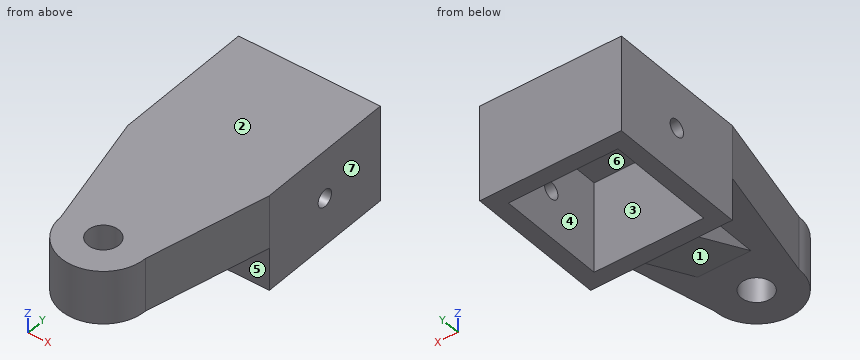
from build123d import *

# Parameters (mm, degrees)
CROQUIS1_W                   = 26.5
CROQUIS1_H                   = 26.5
CROQUIS1_W_2                 = 20.5
CROQUIS1_H_2                 = 20.5
SALIENTE_EXTRUIR1_DEPTH      = 9
SALIENTE_EXTRUIR2_DEPTH      = 9
SALIENTE_EXTRUIR2_DEPTH_BACK = 1
CROQUIS2_R                   = 2.9
CROQUIS5_W                   = 20.5
CROQUIS5_H                   = 20.5
SALIENTE_EXTRUIR3_DEPTH      = 1
NERVIO6_REACH                = 48.731
CROQUIS3_WALL_W              = 111.809486112
CROQUIS3_WALL_H              = 10
CROQUIS4_R                   = 1.6
CORTAR_EXTRUIR2_DEPTH        = 25


with BuildPart() as part:
    # Croquis1 → Saliente-Extruir1 (new, symmetric)
    with BuildSketch(Plane.XY):
        Rectangle(CROQUIS1_W, CROQUIS1_H)
        Rectangle(CROQUIS1_W_2, CROQUIS1_H_2, mode=Mode.SUBTRACT)
    extrude(amount=SALIENTE_EXTRUIR1_DEPTH, both=True)

    # Croquis2 → Saliente-Extruir2 (add, two sides: drawn at the far end of the back side and taken through both)
    with BuildSketch(Plane.XY.offset(-SALIENTE_EXTRUIR2_DEPTH_BACK)):
        with BuildLine():
            Line((-7.9, -36), (-13.25, -13.25))
            Line((-13.25, -13.25), (13.25, -13.25))
            Line((13.25, -13.25), (7.9, -36))
            ThreePointArc((7.9, -36), (0, -43.9), (-7.9, -36))
        make_face()
        with Locations((0, -36)):
            Circle(CROQUIS2_R, mode=Mode.SUBTRACT)
    extrude(amount=SALIENTE_EXTRUIR2_DEPTH + SALIENTE_EXTRUIR2_DEPTH_BACK)

    # Croquis5 → Saliente-Extruir3 (add)
    with BuildSketch(Plane.XY.offset(9)):
        Rectangle(CROQUIS5_W, CROQUIS5_H)
    extrude(amount=-SALIENTE_EXTRUIR3_DEPTH)

    # Croquis3 wall → Nervio6 (add, up to next)
    with BuildSketch(Plane(origin=(0, -20.75, -4.25), x_dir=(0, 0.91755562531, -0.397607437634), z_dir=(0, 0.397607437634, 0.91755562531)), mode=Mode.PRIVATE) as nervio6_sk1:
        Rectangle(CROQUIS3_WALL_W, CROQUIS3_WALL_H)
    nervio6_tool1 = extrude(nervio6_sk1.sketch, amount=NERVIO6_REACH, mode=Mode.PRIVATE) - part.part
    add(nervio6_tool1.solids().sort_by_distance((0, -20.75, -4.25))[0])

    # Croquis4 → Cortar-Extruir2 (cut, symmetric)
    with BuildSketch(Plane(origin=(0, 0, 0), x_dir=(0, 0, -1), z_dir=(1, 0, 0))):
        Circle(CROQUIS4_R)
    extrude(amount=CORTAR_EXTRUIR2_DEPTH, both=True, mode=Mode.SUBTRACT)


solid = part.part
The listing builds one solid part. Answer for the finished solid, in the listing's coordinates (mm). Face numbers are marked on the shaded views. A direction names the side the tool comes from. Give positions to 0.01 mm unless a question says otherwise; leave off trailing zeros. Order: outer loops, then holes, each group sorted by start corner. A loop starts at its lowest first (then second) coordinate and runs counter-clockwise, first axis right, second up. Notation, with made-up numbers: (35.25, 80) - (60.25, 80) arc R34 ccw to (60.25, 119) - close; hole circle Ø1 at (49, 73). An arc over 180 degrees is marked (long way). One line per item, written item: value. Start each with the question number.
1) A cutting plane is placed at B-B on x = 0. Give the vertices of the cut face in (y, z), then the cut area to 3 significant figures.
2) A cutting plane is placed at A-A on z = 0. Give the vertices of the cut face in (x, y), then the cut area to 3 significant figures.
3) Given pin 1 Ø7 at (y, z) = (-24.5, -2.5) entering from +X; pin 2 Ø1.5 at (x, z) = (-5, 1) entering from -Y; pin 3 Ø5 at (y, z) = (-18, 6) entering from +X, each flat-ended and moving along its own axis, determine where each tip first touches the part or whether it passes through.
4) A tool of negligible diameter and unlimited length cuts with its end or side. For the marked faces 5, 6 and 7, from which of +Z, -Z, +X, -X, +Y, -Y can it reach the whole face along a straight path? Write none if from no direction.
5) A cutting plane is placed at C-C on y = 0. Give the vertices of the cut face in (x, z), then the cut area to 3 significant figures.
6) The mould has two halves that part along Y. Classify the marked faces 1, 2, 3 and 4: released by +Y, released by -Y, zero draft, split by the parting line, or undercut.
7) A cutting plane is placed at D-D on z = 7. Give the vertices of the cut face in (x, y).
8) Find the intervals of material crossed by L1, parallel to Y at x = -8.25, z = -5.5; L2, parallel to Y at x = -4.75, z = 5, in increasing order.
Answer sheet:
1. outline: (-43.9, -1) - (-38.9, -1) - (-38.9, 9) - (-43.9, 9) - close; (-33.1, -1) - (-28.25, -1) - (-13.25, -7.5) - (-13.25, -9) - (-10.25, -9) - (-10.25, 8) - (10.25, 8) - (10.25, -9) - (13.25, -9) - (13.25, 9) - (-33.1, 9) - close
1. area: 426 mm2
2. outline: (-13.25, -13.25) - (-7.9, -36) arc R7.9 ccw to (7.9, -36) - (13.25, -13.25) - (13.25, -1.6) - (10.25, -1.6) - (10.25, -10.25) - (-10.25, -10.25) - (-10.25, -1.6) - (-13.25, -1.6) - close; (-13.25, 1.6) - (-10.25, 1.6) - (-10.25, 10.25) - (10.25, 10.25) - (10.25, 1.6) - (13.25, 1.6) - (13.25, 13.25) - (-13.25, 13.25) - close; hole circle Ø5.8 at (0, -36)
2. area: 816 mm2
3. pin 1: stops at x = 11.35
3. pin 2: stops at y = -42.66
3. pin 3: stops at x = 12.72
4. face 5: -Z, -Y
4. face 6: -Z
4. face 7: +Z, -Z, +X, +Y, -Y
5. outline: (-13.25, -9) - (-10.25, -9) - (-10.25, -1.6) - (-13.25, -1.6) - close; (-13.25, 1.6) - (-10.25, 1.6) - (-10.25, 8) - (10.25, 8) - (10.25, 1.6) - (13.25, 1.6) - (13.25, 9) - (-13.25, 9) - close; (10.25, -9) - (13.25, -9) - (13.25, -1.6) - (10.25, -1.6) - close
5. area: 109 mm2
6. face 1: released by -Y
6. face 2: zero draft
6. face 3: undercut
6. face 4: undercut
7. outline: (-13.25, -13.25) - (-7.9, -36) arc R7.9 ccw to (7.9, -36) - (13.25, -13.25) - (13.25, 13.25) - (-13.25, 13.25) - close; hole (-10.25, -10.25) - (10.25, -10.25) - (10.25, 10.25) - (-10.25, 10.25) - close; hole circle Ø5.8 at (0, -36)
8. L1: y = -13.25 to -10.25, 10.25 to 13.25
8. L2: y = -42.31 to -10.25, 10.25 to 13.25
